```python
from build123d import *

# Parameters (mm, degrees)
F0_R     = 63.5
F0_W     = 25.4
F0_H     = 25.4
F1_DEPTH = 50.8
F2_DEPTH = 50.8


with BuildPart() as f1:
    # F0 (on Front) → F1 (new body)
    with BuildSketch(Plane.XZ):
        Circle(F0_R)
        Rectangle(F0_W, F0_H, mode=Mode.SUBTRACT)
    extrude(amount=F1_DEPTH)

    # F0 (on Front) → F2 (join)
    with BuildSketch(Plane.XZ):
        Circle(F0_R)
        Rectangle(F0_W, F0_H, mode=Mode.SUBTRACT)
    extrude(amount=-F2_DEPTH)


solid = f1.part
```
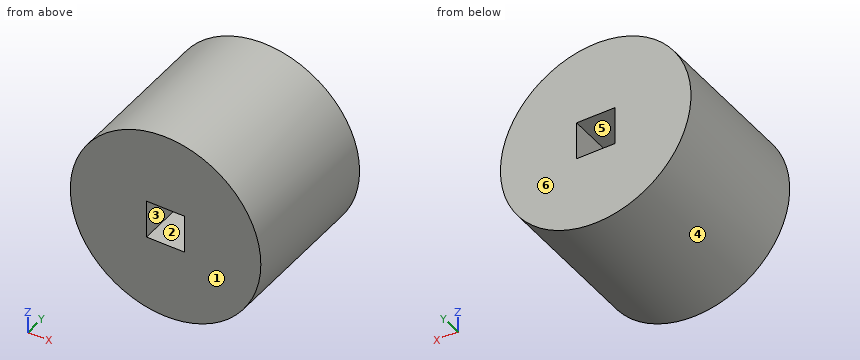
Geometry: final body of the model. Coordinates: model frame, mm. Face numbers are marked on the shaded views. A direction names the side the tool comes from. Round coordinates to 2 decimals unless told otherwise and drop trailing zeros. Order: outer loops, then holes, each group sorted by start corner. A loop starts at its lowest first (then second) coordinate and runs counter-clockwise, first axis right, second up. Notation, with made-up numbers: M -37,61.25 L -5,61.25 A14 ccw -5,76.25 Z; hole C 83,29 d6. An arc over 180 degrees is marked long. One line per item, written item: value.
(1) Cut plane C-C (y = -38). Return the cut outline in (x, z), and give its area (3 significant figures).
Result sheet:
outline: C 0,0 d127; hole M -12.7,-12.7 L 12.7,-12.7 L 12.7,12.7 L -12.7,12.7 Z
area: 12,000 mm2
(2) Pull-direction query (Z, two-part tool) for the marked faces 3, 4, 5 and 6; classes: pulls with the +Z half, pulls with the -Z half, needs draft (parallel to the pull), parting line crosses it, or undercut.
Result sheet:
face 3: undercut
face 4: parting line crosses it
face 5: undercut
face 6: needs draft
(3) Cut plane D-D (z = -17.5). Return the cut outline in (x, y), and give its area (3 significant figures).
Result sheet:
outline: M -61.04,-50.8 L 61.04,-50.8 L 61.04,50.8 L -61.04,50.8 Z
area: 12,400 mm2
(4) Line query: probe 1 along X at (y, z) = (24, 1); probe 2 along X at (y, z) = (-11, -10); probe 3 along Z at (x, y) = (-5, -20). Output: solid intervals per line, ascending. Write a range as [from, to].
Result sheet:
probe 1: [-63.49, -12.7], [12.7, 63.49]
probe 2: [-62.71, -12.7], [12.7, 62.71]
probe 3: [-63.3, -12.7], [12.7, 63.3]
(5) Cut plane A-A (x = 0). Return the cut outline in (y, z).
Result sheet:
outline: M -50.8,-63.5 L 50.8,-63.5 L 50.8,-12.7 L -50.8,-12.7 Z; M -50.8,12.7 L 50.8,12.7 L 50.8,63.5 L -50.8,63.5 Z
(6) Cut plane B-B (z = 0). Return the cut outline in (x, y), and give its area (3 significant figures).
Result sheet:
outline: M -63.5,-50.8 L -12.7,-50.8 L -12.7,50.8 L -63.5,50.8 Z; M 12.7,-50.8 L 63.5,-50.8 L 63.5,50.8 L 12.7,50.8 Z
area: 10,300 mm2
(7) Reachability of the marked faces 1 and 2 from +Z, -Z, +X, -X, +Y, -Y: full face, straight path, thin tool, end or side. Return the list, or none.
Result sheet:
face 1: +Z, -Z, +X, -X, -Y
face 2: +Y, -Y
(8) Pin query (flat end, axial travel): P1, Ø2, axis at y = 5.5, z = -38.5, coming from the +X side; P2, Ø5, axis at y = -4.5, z = 15.5, coming from the -X side; P3, Ø1, axis at y = -5, z = -41, coming from the +X side. Return the tip coordinate at first contact, or that it passes through.
Result sheet:
P1: x = 51.24
P2: x = -62.16
P3: x = 48.91
